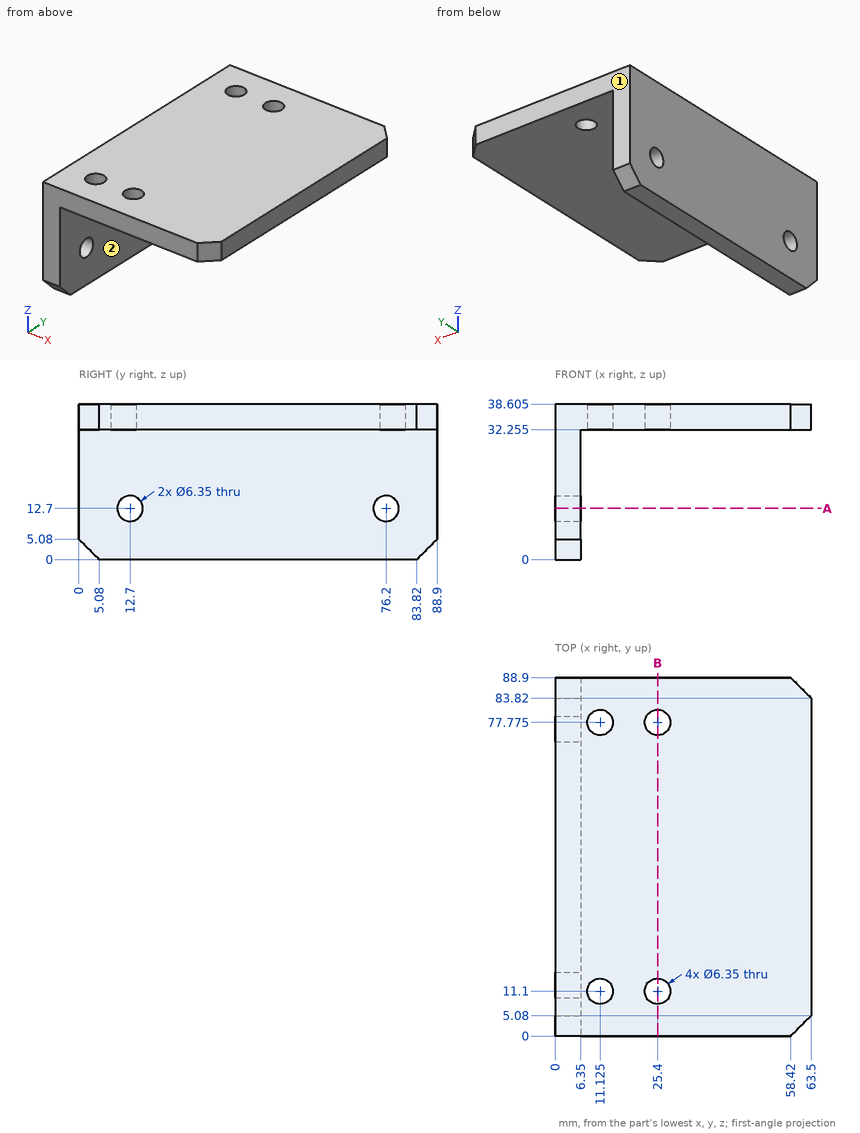
Can you work these out from the drawing? Everything is in mm from the part's minimum corner. A direction names the side the tool comes from. Coordinates: 2 decimals unless noted, no trailing zeros. Loops run counter-clockwise (first coordinate to the right, second up) from the corner with the lowest first, then second, coordinate; pieces in that order, holes last.
1) Which directions (+Z, -Z, +X, -X, +Y, -Y) give clear straight access to the entire face, cutting with the end or side of a thin tool? Please do the marked faces 1 and 2.
Reported:
face 1: +Z, -Z, +X, -X, +Y
face 2: -Z, +X, +Y, -Y
2) Will these pins go through, and if not, where does the flat tip stop? pin 1 Ø1.5 at (y, z) = (26, 23.5) entering from +X; pin 2 Ø7.5 at (x, y) = (25.4, 11.1) entering from -Z (3 decimals).
Reported:
pin 1: stops at x = 6.35
pin 2: stops at z = 32.255
3) Imagine slicing it at B-B (x = 25.4). State how many separate pieces and enclosed holes the cut face has, and give its area (3 significant figures).
Reported:
separate pieces: 3
enclosed holes: 0
area: 484 mm2
4) Please list where these lines run through material, in increasing order: line 1 along Y through (x, z) = (1, 12); line 2 along Z through (x, y) = (58, 9) (1 decimal); line 3 along X through (y, z) = (25, 30.5).
Reported:
line 1: y = 0 to 9.6, 15.8 to 73.1, 79.3 to 88.9
line 2: z = 32.3 to 38.6
line 3: x = 0 to 6.35
5) Imagine slicing it at A-A (z = 12.7). List the corners of the cut face in (x, y) for me (3 decimals).
Reported:
outline: (0, 0) - (6.35, 0) - (6.35, 9.525) - (0, 9.525) - close; (0, 15.875) - (6.35, 15.875) - (6.35, 73.025) - (0, 73.025) - close; (0, 79.375) - (6.35, 79.375) - (6.35, 88.9) - (0, 88.9) - close
